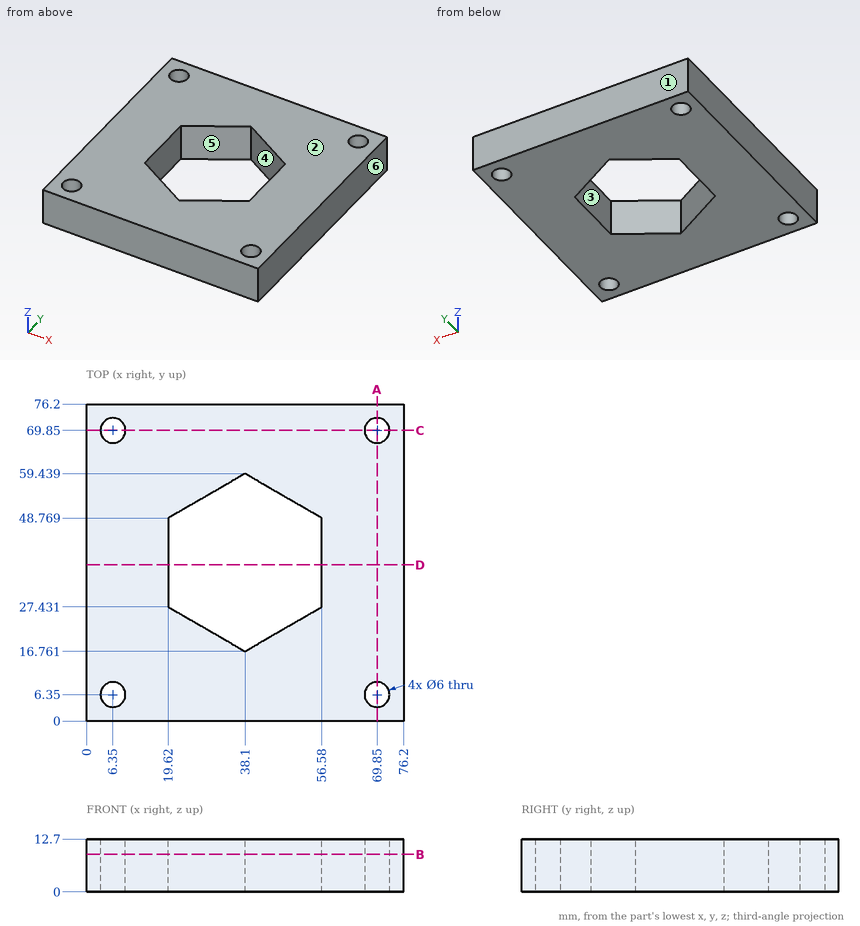
Study the drawing (mm; zero at the part's minimum x, y, z) and answer. A direction names the side the tool comes from. Give positions to 0.01 mm unless a question says otherwise; leave off trailing zeros. Write each loop counter-clockwise with the first axis right and the second up, starting at its lowest first coordinate (ties: lowest second). Pieces come first, ordered by that corner, then holes. Notation, with made-up numbers: (-7, 2.25) - (49, 2.25) arc R32 ccw to (49, 33.25) - close; hole circle Ø2 at (-26.5, 32). An arc over 180 degrees is marked (long way). Write item = value, one per line. Start each with the question number.
Item 1: A tool of negligible diameter and unlimited length cuts with its end or side. For the marked faces 5 and 6, from which of +Z, -Z, +X, -X, +Y, -Y can it reach the whole face along a straight path? Write none if from no direction.
Item 2: Find the intervals of material crossed by probe 1 along X at (y, z) = (47, 11.5); probe 2 along Y at (x, z) = (69.85, 2.5); probe 3 along Y at (x, z) = (69, 8), in increasing order. Write a range as [from, to].
Item 3: Find section A-A (x = 69.85). Give the vertices of the cut face in (y, z).
Item 4: Find section D-D (y = 37.5). Give the vertices of the cut face in (x, z).
Item 5: Find section B-B (z = 9). Give the vertices of the cut face in (x, y).
Item 6: This flat-tipped pin is pushed along its axis until it touches: P1, Ø8, axis at x = 6.35, y = 6.35, coming from the -Z side. Where does it stop, or does it pass through?
Item 7: The mould has two halves that part along Y. Classify the marked faces 1, 2, 3 and 4: +Y half, -Y half, draft (parallel to the pull), parting line (faces both ways), or undercut.
Response:
q1.face_5 = +Z, -Z
q1.face_6 = +Z, -Z, +X, +Y, -Y
q2.probe_1 = [0, 19.62], [56.58, 76.2]
q2.probe_2 = [0, 3.35], [9.35, 66.85], [72.85, 76.2]
q2.probe_3 = [0, 3.47], [9.23, 66.97], [72.73, 76.2]
q3.outline = (0, 0) - (3.35, 0) - (3.35, 12.7) - (0, 12.7) - close; (9.35, 0) - (66.85, 0) - (66.85, 12.7) - (9.35, 12.7) - close; (72.85, 0) - (76.2, 0) - (76.2, 12.7) - (72.85, 12.7) - close
q4.outline = (0, 0) - (19.62, 0) - (19.62, 12.7) - (0, 12.7) - close; (56.58, 0) - (76.2, 0) - (76.2, 12.7) - (56.58, 12.7) - close
q5.outline = (0, 0) - (76.2, 0) - (76.2, 76.2) - (0, 76.2) - close; hole circle Ø6 at (6.35, 6.35); hole circle Ø6 at (6.35, 69.85); hole (19.62, 27.43) - (38.1, 16.76) - (56.58, 27.43) - (56.58, 48.77) - (38.1, 59.44) - (19.62, 48.77) - close; hole circle Ø6 at (69.85, 6.35); hole circle Ø6 at (69.85, 69.85)
q6.P1 = 0
q7.face_1 = +Y half
q7.face_2 = draft
q7.face_3 = undercut
q7.face_4 = undercut
